Build history of the part. All positions in model axes, mm. A direction names the side the tool comes from. Round coordinates to 2 decimals unless told otherwise and drop trailing zeros. Write each loop counter-clockwise with the first axis right and the second up, starting at its lowest first coordinate (ties: lowest second). Pieces come first, ordered by that corner, then holes. Notation, with made-up numbers: (62.25, 68.25) -> (104.25, 68.25) arc R23 ccw to (104.25, 89.25) -> close; hole circle Ø11 at (1, 76.25). An arc over 180 degrees is marked (long way). Answer as CSV lines item,"result".
from build123d import *

# Parameters (mm, degrees)
BOSS_EXTRUDE1_DEPTH = 36
SKETCH2_R           = 4.5
CUT_EXTRUDE1_DEPTH  = 30
SKETCH3_R           = 2.5
CUT_EXTRUDE2_DEPTH  = 10


with BuildPart() as part:
    # Sketch1 → Boss-Extrude1 (new body)
    with BuildSketch(Plane.XY):
        Polygon((-123.814545152, -26.546784039), (-43.814545152, -26.546784039), (-43.814545152, -15.688919663), (-43.814545152, -8), (-29.603926395, -8), (0.496524767, -8), (36.185454848, -8), (36.185454848, 0), (-33.18939726, 0), (-55.814545152, 0), (-55.814545152, -18.546784039), (-123.814545152, -18.546784039), align=None)
    extrude(amount=BOSS_EXTRUDE1_DEPTH)

    # Sketch2 → Cut-Extrude1 (cut)
    with BuildSketch(Plane(origin=(0, 0, 0), x_dir=(1, 0, 0), z_dir=(0, 1, 0))):
        with Locations(Location((24.611399957, -18, 0), (0, 0, 180))):
            Circle(SKETCH2_R)
    extrude(amount=-CUT_EXTRUDE1_DEPTH, mode=Mode.SUBTRACT)

    # Sketch3 → Cut-Extrude2 (cut)
    with BuildSketch(Plane(origin=(0, -18.546784039, 0), x_dir=(1, 0, 0), z_dir=(0, 1, 0))):
        with Locations(Location((-108.814545152, -18, 0), (0, 0, 270))):
            Circle(SKETCH3_R)
        with Locations(Location((-70.814545152, -18, 0), (0, 0, 270))):
            Circle(SKETCH3_R)
    extrude(amount=-CUT_EXTRUDE2_DEPTH, mode=Mode.SUBTRACT)


solid = part.part
1. Which spindle directions (+Z, -Z, +X, -X, +Y, -Y) get a long thin tool onto all of the face, cutting with end or side? Do faces 4 (the cylindrical face through (-111.255, -22.491, 17.458)), 5 (the flat face through (-4, -8, 18)), 6 (the flat face through (-89, -18.547, 18)). Say none if no direction does.
Results found:
face 4,"+Y, -Y"
face 5,"+Z, -Z, +X, -Y"
face 6,"+Z, -Z, -X, +Y"
2. Mould opens along X. For faces 1 (the cylindrical face through (27.93, -3.94, 21.04)), 2 (the flat face through (-9, 0, 18)), 3 (the flat face through (-123.815, -22, 18)) say: +X half, -X half, draft (parallel to the pull), parting line (faces both ways), or undercut.
Results found:
face 1,"undercut"
face 2,"draft"
face 3,"-X half"
3. Cut at D-D, the plane y = -25. Write the cut outline in (x, z), then the cut area to 3 significant figures.
Results found:
outline,"(-123.81, 0) -> (-43.81, 0) -> (-43.81, 36) -> (-123.81, 36) -> close; hole circle Ø5 at (-108.81, 18); hole circle Ø5 at (-70.81, 18)"
area,"2,840 mm2"
4. Cut at B-B, the plane y = -4. Write the cut outline in (x, z), then the cut area to 3 significant figures.
Results found:
outline,"(-55.81, 0) -> (36.19, 0) -> (36.19, 36) -> (-55.81, 36) -> close; hole circle Ø9 at (24.61, 18)"
area,"3,250 mm2"
5. Drop flat-ended pins along their axis: pin 1 Ø1.5 at (x, z) = (-20, 12) entering from -Y; pin 2 Ø4 at (x, z) = (-108.81, 18) entering from -Y; pin 3 Ø9.5 at (y, z) = (-14.5, 26) entering from +X; pin 4 Ø18 at (x, z) = (-85.5, 24) entering from +Y. Give the stop position or say it passes through.
Results found:
pin 1,"stops at y = -8"
pin 2,"passes through"
pin 3,"stops at x = -43.81"
pin 4,"stops at y = -18.55"
6. Cut at A-A, the plane z = 18. Write the cut outline in (x, y).
Results found:
outline,"(-123.81, -26.55) -> (-111.31, -26.55) -> (-111.31, -18.55) -> (-123.81, -18.55) -> close; (-106.31, -26.55) -> (-73.31, -26.55) -> (-73.31, -18.55) -> (-106.31, -18.55) -> close; (-68.31, -26.55) -> (-43.81, -26.55) -> (-43.81, -8) -> (20.11, -8) -> (20.11, 0) -> (-55.81, 0) -> (-55.81, -18.55) -> (-68.31, -18.55) -> close; (29.11, -8) -> (36.19, -8) -> (36.19, 0) -> (29.11, 0) -> close"
7. Probe line 1 along X through (y, z) = (-23.5, 18); line 2 along X through (y, z) = (-24.25, 19); line 3 along Y through (x, z) = (-110.5, 21.5). List the from-to ranges inside material, lowest first.
Results found:
line 1,"x = -123.81 to -111.31, -106.31 to -73.31, -68.31 to -43.81"
line 2,"x = -123.81 to -111.11, -106.52 to -73.11, -68.52 to -43.81"
line 3,"y = -26.55 to -18.55"
8. Cut at C-C, the plane z = 24. Write the cut outline in (x, y), then the cut area to 3 significant figures.
Results found:
outline,"(-123.81, -26.55) -> (-43.81, -26.55) -> (-43.81, -8) -> (36.19, -8) -> (36.19, 0) -> (-55.81, 0) -> (-55.81, -18.55) -> (-123.81, -18.55) -> close"
area,"1,500 mm2"
